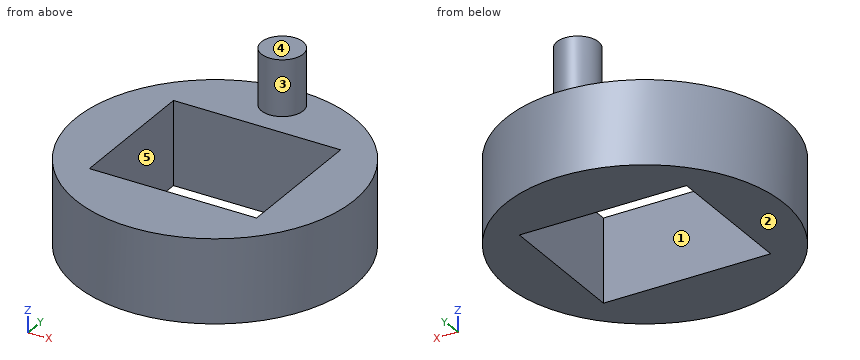
Autodesk Fusion 360 part; units mm, degrees
sketch "Sketch1" plane through (0, 0, 0) normal (0, 0, 1) x (1, 0, 0)
  circle A0 centre (0, 0) radius 50
  dimension "d1" = 100
extrude "Extrude1" add sketch "Sketch1" along normal blind 30
sketch "Sketch2" plane through (0, 0, 30) normal (0, 0, 1) x (-1, 0, 0)
  circle A0 centre (0, 0) radius 50
  line L0 (30, 25) -> (-30, 25)
  line L1 (-30, 25) -> (-30, -25)
  line L2 (-30, -25) -> (30, -25)
  line L3 (30, -25) -> (30, 25)
  line L4 (30, 25) -> (-30, -25) construction
  line L5 (-30, 25) -> (30, -25) construction
  dimension "d4" = 60
  dimension "d5" = 50
extrude "Extrude2" cut sketch "Sketch2" against normal blind 30 contours L0 L1 L2 L3
sketch "Sketch3" plane through (0, 0, 30) normal (0, 0, 1) x (-1, 0, 0)
  line L0 (-30, 25) -> (30, 25)
  line L1 (30, 25) -> (30, -25)
  line L2 (30, -25) -> (-30, -25)
  line L3 (-30, -25) -> (-30, 25)
  circle A0 centre (0, 0) radius 50
  circle A1 centre (0, -40) radius 7.5
  dimension "d8" = 15
extrude "Extrude3" add sketch "Sketch3" along normal blind 20 contours A1
Check sheet for the modelled part. Datum: model origin and axes. Units: mm. Face numbers are marked on the shaded views. A direction names the side the tool comes from. Give positions to 0.01 mm unless a question says otherwise; leave off trailing zeros. Write each loop counter-clockwise with the first axis right and the second up, starting at its lowest first coordinate (ties: lowest second). Pieces come first, ordered by that corner, then holes. Notation, with made-up numbers: (-3, -21.5) - (5, -21.5) arc R16 cw to (5, -2.5) - close; hole circle Ø11 at (-30.5, 13.5). An arc over 180 degrees is marked (long way). Answer as a JSON object with one key per item and string values. Group by question number.
1) Sectioned sample at A-A (x = 0). Record the cut outline in (y, z), then the cut area to 3 significant figures.
2) Thickness scan on probe 1 along Y at (x, z) = (1.5, 24.5); probe 2 along X at (y, z) = (-1, 29.5); probe 3 along Z at (x, y) = (-40.5, -6). Record the ranges inside material, lowest first. Write a range as from..to.
3) Depth check by flat-ended pin: P1, Ø10, axis at y = 8.5, z = 16, coming from the -X side; P2, Ø15, axis at x = -10.5, z = 14.5, coming from the +Y side; P3, Ø1.5, axis at y = 31, z = 13, coming from the +X side. Enter the tip coordinate at first touch or a pass-through.
4) Sectioned sample at D-D (y = 40). Record the cut outline in (x, z).
5) Access from +Z, -Z, +X, -X, +Y, -Y to the whole of each face (thin tool, end or side, straight path). Record for the marked faces 1 and 2.
6) Sectioned sample at B-B (y = 0). Record the cut outline in (x, z).
7) Sectioned sample at C-C (z = 23). Record the cut outline in (x, y), then the cut area to 3 significant figures.
8) Release check for a two-part mould opening along X. For the marked faces 3, 4 and 5 record: pulls with the +X half, pulls with the -X half, needs draft (parallel to the pull), parting line crosses it, or undercut.
Geometry results:
{
 "1": {"outline": "(-50, 0) - (-25, 0) - (-25, 30) - (-50, 30) - close; (25, 0) - (50, 0) - (50, 30) - (47.5, 30) - (47.5, 50) - (32.5, 50) - (32.5, 30) - (25, 30) - close", "area": "1,800 mm^2"},
 "2": {"probe 1": "y = -49.98..-25, 25..49.98", "probe 2": "x = -49.99..-30, 30..49.99", "probe 3": "z = 0..30"},
 "3": {"P1": "stops at x = -49.88", "P2": "stops at y = 49.91", "P3": "stops at x = 39.81"},
 "4": {"outline": "(-30, 0) - (30, 0) - (30, 30) - (7.5, 30) - (7.5, 50) - (-7.5, 50) - (-7.5, 30) - (-30, 30) - close"},
 "5": {"face 1": "+Z, -Z", "face 2": "-Z, +X, -X, +Y, -Y"},
 "6": {"outline": "(-50, 0) - (-30, 0) - (-30, 30) - (-50, 30) - close; (30, 0) - (50, 0) - (50, 30) - (30, 30) - close"},
 "7": {"outline": "circle Ø100 at (0, 0); hole (-30, -25) - (30, -25) - (30, 25) - (-30, 25) - close", "area": "4,850 mm^2"},
 "8": {"face 3": "parting line crosses it", "face 4": "needs draft", "face 5": "undercut"}
}
